Autodesk Inventor part; units mm, degrees
ref_plane "Plan de construction2" through (0, 6, 2) normal (0, 1, 0) x (1, 0, 0)
ref_plane "YZ Plane" through (0, 0, 0) normal (1, 0, 0) x (0, 1, 0)
ref_plane "XZ Plane" through (0, 0, 0) normal (0, 1, 0) x (-1, 0, 0)
sketch "Esquisse1" plane through (0, 0, 0) normal (0, 0, 1) x (1, 0, 0)
  line L0 (0, 0) -> (8, 0)
  line L1 (8, 0) -> (8, 12)
  line L2 (8, 12) -> (0, 12)
  line L3 (0, 12) -> (0, 0)
  dimension "d0" = 8
  dimension "d1" = 12
extrude "Extrusion1" add sketch "Esquisse1" along normal blind 2
sketch "Esquisse2" plane through (0, 0, 2) normal (0, 0, 1) x (1, 0, 0)
  line L0 (8, 0) -> (8, 12)
  line L1 (8, 12) -> (18, 12)
  line L2 (18, 12) -> (18, 0)
  line L3 (18, 0) -> (8, 0)
  line L4 (8, 0) -> (8, 12)
  point P0 (0, 0)
  dimension "d7" = 10
extrude "Extrusion2" add sketch "Esquisse2" against normal blind 7
chamfer "Chanfrein1" distance 5 distance2 8 1 edges at (8, 6, 0) measured on face at (8, 4, -1.6667)
sketch "Esquisse3" plane through (0, 0, -5) normal (0, 0, -1) x (-1, 0, 0)
  arc A0 (-4, 10) -> (-4, 2) centre (-4, 6) ccw
  line L0 (-8, 0) -> (-8, 12)
  line L1 (-4, 2) -> (4, 2)
  line L2 (4, 2) -> (4, 10)
  line L3 (4, 10) -> (-4, 10)
  point P0 (0, 0)
  dimension "d13" = 8
extrude "Extrusion3" cut sketch "Esquisse3" against normal blind 5
sketch "Esquisse4" plane through (0, 0, 0) normal (0, 0, -1) x (-1, 0, 0)
  arc A0 (-4, 10) -> (-8, 6) centre (-4, 6) ccw
  circle A1 centre (-4, 6) radius 2.1
  point P0 (0, 0)
  dimension "d16" = 4.2
extrude "Extrusion4" cut sketch "Esquisse4" against normal through all
ref_plane "Plan de construction2" through (0, 6, 2) normal (0, 1, 0) x (1, 0, 0)
sketch "Esquisse10" plane through (0, 6, 2) normal (0, 1, 0) x (1, 0, 0)
  line L0 (18, 7) -> (8, 7)
  circle A0 centre (13, 7) radius 3.5
  point P0 (0, 2)
  dimension "d29" = 7
sketch "Esquisse12" plane through (0, 0, -5) normal (0, 0, -1) x (-1, 0, 0)
  line L0 (-9.5, 6) -> (-16.5, 6)
  line L1 (-8.5, 11) -> (-10.5, 11)
  line L2 (-10.5, 11) -> (-10.5, 1)
  line L3 (-10.5, 1) -> (-8.5, 1)
  line L4 (-8.5, 1) -> (-8.5, 11)
  line L5 (-8.5, 11) -> (-10.5, 1) construction
  line L6 (-10.5, 11) -> (-8.5, 1) construction
  point P0 (0, 0)
  dimension "d30" = 2
sweep "Balayage2" cut profiles "Esquisse12" path "Esquisse10" path curves A0
sketch "Esquisse13" plane through (0, 6, 2) normal (0, 1, 0) x (1, 0, 0)
  line L0 (8, 7) -> (18, 7)
  circle A0 centre (13, 7) radius 1.5
  point P0 (0, 2)
  dimension "d33" = 3
extrude "Extrusion6" cut sketch "Esquisse13" along normal through all both and the other way through all
fillet "Congé3" radius 1 4 edges at (14.5, 3, -5) (14.5, 9, -5) (11.5, 9, -5) (11.5, 3, -5)
fillet "Congé4" radius 1 4 edges at (18, 12, -1.5) (18, 0, -1.5) (0, 0, 1) (0, 12, 1)
properties part number "passe cable"
Input: part model. Units: mm. Frame: model coordinates. A direction names the side the tool comes from. Coordinates: 2 decimals unless noted, no trailing zeros. Loops run counter-clockwise (first coordinate to the right, second up) from the corner with the lowest first, then second, coordinate; pieces in that order, holes last. Notation, with made-up numbers: (61, 22) -> (96, 22) arc R20 ccw to (96, 50) -> close; hole circle Ø2 at (27, 29.25). An arc over 180 degrees is marked (long way). Write each question's results on one line, items separated by ' | '. Start each with the question number.
Q1. Section C-C, the plane y = 5.75. State how many separate pieces and enclosed holes the cut face has, plus the area to 3 significant figures.
Q2. Ray query, line 1 (Y direction, x = 4, z = 1.55); line 2 (Z direction, x = 5, y = 3.25); line 3 (X direction, y = 9, z = -1.75). Return the intervals inside material, ascending. Write a range as from..to.
Q3. Pin query (flat end, axial travel): pin 1 (6.5 mm diameter, centred on x = 2.5, y = 8.5, fed in from -Z). Return the tip coordinate at first contact, or that it passes through.
Q4. Section A-A, the plane z = 1.25. Return the cut outline in (x, y), plus the area to 3 significant figures.
Q5. Pull-direction query (Y, two-part tool) for faces 6 (the flat face through (2, 2, -1)), 7 (the cylindrical face through (14.737, 5.916, -4.832)), 8 (the cylindrical face through (8, 6, -2)), 9 (the cylindrical face through (0.285, 0.301, 0.998)); classes: released by +Y, released by -Y, zero draft, split by the parting line, or undercut.
Q6. Reachability of faces 1 (the flat face through (18, 6, -1)), 2 (the cylindrical face through (12.9, 6.1, -0.5)), 3 (the cylindrical face through (11.25, 5.92, -4.84)), 4 (the flat face through (9, 12, -1)), 5 (the flat face through (1, 6, 0)) from +Z, -Z, +X, -X, +Y, -Y: full face, straight path, thin tool, end or side. Return the list, or none.
Found:
1) separate pieces: 3 | enclosed holes: 0 | area: 52.0 mm2
2) line 1: 0..3.9, 8.1..12 | line 2: 0..2 | line 3: 6.65..9.89, 16.11..18
3) pin 1: z = -3.45
4) outline: (0, 1) arc R1 ccw to (1, 0) -> (17, 0) arc R1 ccw to (18, 1) -> (18, 11) arc R1 ccw to (17, 12) -> (1, 12) arc R1 ccw to (0, 11) -> close; hole circle Ø4.2 at (4, 6) | area: 201 mm2
5) face 6: undercut | face 7: zero draft | face 8: undercut | face 9: released by -Y
6) face 1: +Z, -Z, +X, +Y, -Y | face 2: none | face 3: -Z, +Y, -Y | face 4: +Z, -Z, +X, -X, +Y | face 5: -Z, -X
